The listing builds one solid part. Answer for the finished solid, in the listing's coordinates (mm). Round coordinates to 2 decimals unless told otherwise and drop trailing zeros. Write each loop counter-clockwise with the first axis right and the second up, starting at its lowest first coordinate (ties: lowest second). Pieces come first, ordered by that corner, then holes. Notation, with made-up numbers: (40.5, 33.25) -> (55.5, 33.25) arc R21 ccw to (55.5, 66.25) -> close; hole circle Ø8 at (-20, 56). An arc over 180 degrees is marked (long way). Write each question's results on one line, items separated by ' | '. Start each with the question number.
```python
from build123d import *

# Parameters (mm, degrees)
F0_R          = 29
F0_R_2        = 24.2
F1_DEPTH      = 75
F2_R          = 29
F2_R_2        = 24.2
F3_DEPTH      = 29
F3_DEPTH_BACK = 29
F4_R          = 24.2
F5_DEPTH      = 58.001


with BuildPart() as f1:
    # F0 (on Front) → F1 (new body)
    with BuildSketch(Plane.XZ):
        Circle(F0_R)
        Circle(F0_R_2, mode=Mode.SUBTRACT)
    extrude(amount=F1_DEPTH)

    # F2 (on Top) → F3 (join, two sides)
    with BuildSketch(Plane.XY) as f3_sk:
        with Locations((0, 10)):
            Circle(F2_R)
        with Locations((0, 10)):
            Circle(F2_R_2, mode=Mode.SUBTRACT)
    extrude(amount=F3_DEPTH)
    extrude(f3_sk.sketch, amount=-F3_DEPTH_BACK)

    # F4 (on face) → F5 (cut, through all)
    with BuildSketch(Plane.XY.offset(29)):
        with Locations((0, 10)):
            Circle(F4_R)
    extrude(amount=-F5_DEPTH, mode=Mode.SUBTRACT)


solid = f1.part
```
Q1. The part is cut by section C-C, the plane y = 23. Write down the section's boundary in (x, z), then the cut area to 3 significant figures.
Q2. Each of these flat-tipped pins is pushed along its axis until it touches: pin 1 (2 mm diameter, centred on x = 22, y = -61, fed in from -Z); pin 2 (4 mm diameter, centred on y = -43.5, z = 20, fed in from -X); pin 3 (1.5 mm diameter, centred on y = 18, z = -6.5, fed in from -X). Where does it stop, or does it pass through?
Q3. The part is cut by section D-D, the plane x = -18.5. Write down the section's boundary in (y, z).
Q4. The part is cut by section B-B, the plane z = 0. Write down the section's boundary in (x, y), then the cut area to 3 significant figures.
Q5. Find the intervals of material crossed by line 1 (Z direction, x = 0, y = -22.5); line 2 (Y direction, x = 1, z = 25.5), in increasing order.
Q6. Determine the mould class of faces 1 (the cylindrical face through (27.66, -45.31, 8.71)), 2 (the flat face through (-6.6, -75, -23.5)), 3 (the cylindrical face through (23.082, -40.007, 7.269)) for opening direction X: pulls with the +X half, pulls with the -X half, needs draft (parallel to the pull), parting line crosses it, or undercut.
Q7. The part is cut by section A-A, the plane y = -8. Write down the section's boundary in (x, z), then the cut area to 3 significant figures.
Answers follow:
1) outline: (-25.92, -29) -> (-20.41, -29) -> (-20.41, 29) -> (-25.92, 29) -> close; (20.41, -29) -> (25.92, -29) -> (25.92, 29) -> (20.41, 29) -> close | area: 639 mm^2
2) pin 1: z = -20 | pin 2: x = -22.74 | pin 3: x = -28.08
3) outline: (-75, -22.33) -> (-12.33, -22.33) -> (-12.33, -29) -> (-5.6, -29) -> (-5.6, 29) -> (-12.33, 29) -> (-12.33, 22.33) -> (-75, 22.33) -> (-75, 15.6) -> (-12.33, 15.6) -> (-12.33, -15.6) -> (-75, -15.6) -> close; (25.6, -29) -> (32.33, -29) -> (32.33, 29) -> (25.6, 29) -> close
4) outline: (-29, -75) -> (-24.2, -75) -> (-24.2, -5.98) arc R29 ccw to (24.2, -5.98) -> (24.2, -75) -> (29, -75) -> (29, 0) -> (27.22, 0) arc R29 ccw (long way) to (-27.22, 0) -> (-29, 0) -> close; hole circle Ø48.4 at (0, 10) | area: 1,500 mm^2
5) line 1: -29 to -24.2, 24.2 to 29 | line 2: -75 to -14.18, 34.18 to 38.98
6) face 1: parting line crosses it | face 2: needs draft | face 3: undercut
7) outline: (-22.74, -29) -> (-16.18, -29) -> (-16.18, 29) -> (-22.74, 29) -> (-22.74, 18) arc R29 ccw to (-22.74, -18) -> close; (16.18, -29) -> (22.74, -29) -> (22.74, -18) arc R29 ccw to (22.74, 18) -> (22.74, 29) -> (16.18, 29) -> close; hole (-22.74, -8.28) -> (-22.74, 8.28) arc R24.2 ccw to start; hole (22.74, -8.28) arc R24.2 ccw to (22.74, 8.28) -> close | area: 1,040 mm^2
